Build history of the part. All positions in model axes, mm. A direction names the side the tool comes from. Coordinates: 2 decimals unless noted, no trailing zeros. Write each loop counter-clockwise with the first axis right and the second up, starting at its lowest first coordinate (ties: lowest second). Pieces come first, ordered by that corner, then holes. Notation, with made-up numbers: (6, -10.75) -> (29, -10.75) arc R27 ccw to (29, 26.25) -> close; hole circle Ø4 at (76, 28). An arc over 180 degrees is marked (long way). Write each question's results on one line, items separated by ' | '. Start each with the question number.
Q1. Drop flat-ended pins along their axis: pin 1 Ø5 at (y, z) = (57, 38.5) entering from -X; pin 2 Ø1.5 at (x, z) = (-61.5, 1.5) entering from +Y; pin 3 Ø1.5 at (y, z) = (22.5, 28.5) entering from +X. Give the stop position or say it passes through.
Q2. Two-plate mould, pull along Z, no slides. Class faces 1 (the face through (-170.096, 39.44, -0.352)), 2 (the face through (147.12, 40.56, 61.2)), 3 (the face through (99, 60, 50)): released by +Z, released by -Z, zero draft, split by the parting line, or undercut.
Q3. Saw through at C-C on z = 6.5. Give the cut face in (x, y), and give its area (3 significant figures).
Q4. Tool access for faces 4 (the face through (-60, 60, 1)), 5 (the face through (-2, 0, -1)): list every direction of +Z, -Z, +X, -X, +Y, -Y with a clear straight run to the whole face (end or side of a thin tool).
Q5. Drill centre lines: line 1 (X direction, y = 71, z = -1); line 2 (X direction, y = 48.5, z = -4); line 3 (Y direction, x = 87, z = -3.5). Where is each one in solid material? Low to high.
Q6. Saw through at A-A on y = 45.5. Give the cut face in (x, z).
Q7. Saw through at D-D on z = 32. Give the cut face in (x, y), and give its area (3 significant figures).
Q8. Saw through at B-B on y = 27.5. Give the cut face in (x, z).
from build123d import *

# Parameters (mm, degrees)
SALIENTE_EXTRUIR1_DEPTH = 80
REDONDEO1_R             = 60
CROQUIS2_W              = 10
CROQUIS2_H              = 100
CORTAR_EXTRUIR1_DEPTH   = 20
CROQUIS3_W              = 5
CROQUIS3_H              = 80
CORTAR_EXTRUIR2_DEPTH   = 40
CROQUIS4_W              = 80
CROQUIS4_H              = 100
CORTAR_EXTRUIR3_DEPTH   = 40


with BuildPart() as part:
    # Croquis1 → Saliente-Extruir1 (new body)
    with BuildSketch(Plane(origin=(0, 0, 0), x_dir=(1, 0, 0), z_dir=(0, 1, 0))):
        with BuildLine():
            Line((-150, -75), (150, -75))
            ThreePointArc((150, -75), (170.096189432, 0), (150, 75))
            Line((150, 75), (-150, 75))
            ThreePointArc((-150, 75), (-170.096189432, 0), (-150, -75))
        make_face()
    extrude(amount=SALIENTE_EXTRUIR1_DEPTH)

    # Redondeo1
    redondeo1_edges = [part.edges().sort_by_distance(p)[0] for p in [
        (150, 40, 75),
        (-150, 40, 75),
        (-150, 40, -75),
        (150, 40, -75),
    ]]
    fillet(redondeo1_edges, radius=REDONDEO1_R)

    # Croquis2 → Cortar-Extruir1 (cut)
    with BuildSketch(Plane(origin=(0, 80, 0), x_dir=(1, 0, 0), z_dir=(0, 1, 0))):
        with Locations((-105, 0)):
            Rectangle(CROQUIS2_W, CROQUIS2_H)
    extrude(amount=-CORTAR_EXTRUIR1_DEPTH, mode=Mode.SUBTRACT)

    # Croquis3 → Cortar-Extruir2 (cut)
    with BuildSketch(Plane(origin=(0, 80, 0), x_dir=(1, 0, 0), z_dir=(0, 1, 0))):
        with Locations((-62.5, 0)):
            Rectangle(CROQUIS3_W, CROQUIS3_H)
    extrude(amount=-CORTAR_EXTRUIR2_DEPTH, mode=Mode.SUBTRACT)

    # Croquis4 → Cortar-Extruir3 (cut)
    with BuildSketch(Plane(origin=(0, 80, 0), x_dir=(1, 0, 0), z_dir=(0, 1, 0))):
        with Locations((100, 0)):
            Rectangle(CROQUIS4_W, CROQUIS4_H)
    extrude(amount=-CORTAR_EXTRUIR3_DEPTH, mode=Mode.SUBTRACT)


solid = part.part
Returned:
1) pin 1: stops at x = -165.04 | pin 2: stops at y = 40 | pin 3: stops at x = 167.47
2) face 1: split by the parting line | face 2: released by +Z | face 3: undercut
3) outline: (-169.96, 0) -> (169.96, 0) -> (169.96, 80) -> (140, 80) -> (140, 40) -> (60, 40) -> (60, 80) -> (-60, 80) -> (-60, 40) -> (-65, 40) -> (-65, 80) -> (-100, 80) -> (-100, 60) -> (-110, 60) -> (-110, 80) -> (-169.96, 80) -> close | area: 23,600 mm2
4) face 4: +Y | face 5: +Z, -Z, +X, -X, -Y
5) line 1: x = -170.09 to -110, -100 to -65, -60 to 60, 140 to 170.09 | line 2: x = -170.04 to -65, -60 to 60, 140 to 170.04 | line 3: y = 0 to 40
6) outline: (-168, -25) arc R60 ccw to (-108.84, -75) -> (108.84, -75) arc R60 ccw to (168, -25) arc R150 ccw to (168, 25) arc R60 ccw to (108.84, 75) -> (-108.84, 75) arc R60 ccw to (-168, 25) arc R150 ccw to start; hole (-65, -40) -> (-60, -40) -> (-60, 40) -> (-65, 40) -> close; hole (60, -50) -> (140, -50) -> (140, 50) -> (60, 50) -> close
7) outline: (-166.38, 0) -> (166.38, 0) -> (166.38, 80) -> (140, 80) -> (140, 40) -> (60, 40) -> (60, 80) -> (-60, 80) -> (-60, 40) -> (-65, 40) -> (-65, 80) -> (-100, 80) -> (-100, 60) -> (-110, 60) -> (-110, 80) -> (-166.38, 80) -> close | area: 23,000 mm2
8) outline: (-168, -25) arc R60 ccw to (-108.84, -75) -> (108.84, -75) arc R60 ccw to (168, -25) arc R150 ccw to (168, 25) arc R60 ccw to (108.84, 75) -> (-108.84, 75) arc R60 ccw to (-168, 25) arc R150 ccw to start
